Geometry check sheet. Reference: drawing and pictorial views, mm from the part's lowest x, y, z. A direction names the side the tool comes from. Give positions to 0.01 mm unless a question says otherwise; leave off trailing zeros. Write each loop counter-clockwise with the first axis right and the second up, starting at its lowest first coordinate (ties: lowest second). Pieces come first, ordered by that corner, then holes. Notation, with made-up numbers: M 29,25 L 46,25 A37 cw 46,61 Z; hole C 60,11.25 d8. An arc over 180 degrees is marked long. Write item = value, one per line. Start each with the question number.
1) Cross-section at D-D, the plane x = 11. Record the cut outline in (y, z), plus the area to 3 significant figures.
2) Cross-section at A-A, the plane x = 6.75. Record the cut outline in (y, z).
3) Cross-section at C-C, the plane y = 35.5. Record the cut outline in (x, z).
4) Access from +Z, -Z, +X, -X, +Y, -Y to the whole of each face (thin tool, end or side, straight path). Record for the marked faces 4 and 5.
5) Scan lines: line 1 along X through (y, z) = (33.5, 1.75); line 2 along Z through (x, y) = (5.75, 25); line 3 along Y through (x, z) = (9.25, 8.5). Record each from-to range of solid material in increasing order. Write a range as [from, to].
6) Mould release check, pull along X, two halves, no side actions. Record for the marked faces 1, 2 and 3: released by +X, released by -X, zero draft, split by the parting line, or undercut.
7) Cross-section at B-B, the plane z = 6.5. Record the cut outline in (x, y), plus the area to 3 significant figures.
8) Go/stop test with a flat-tipped pin: pin 1 (1 mm diameter, centred on x = 1.5, y = 10, fed in from +Z). Record where the tip stops, or that it passes through.
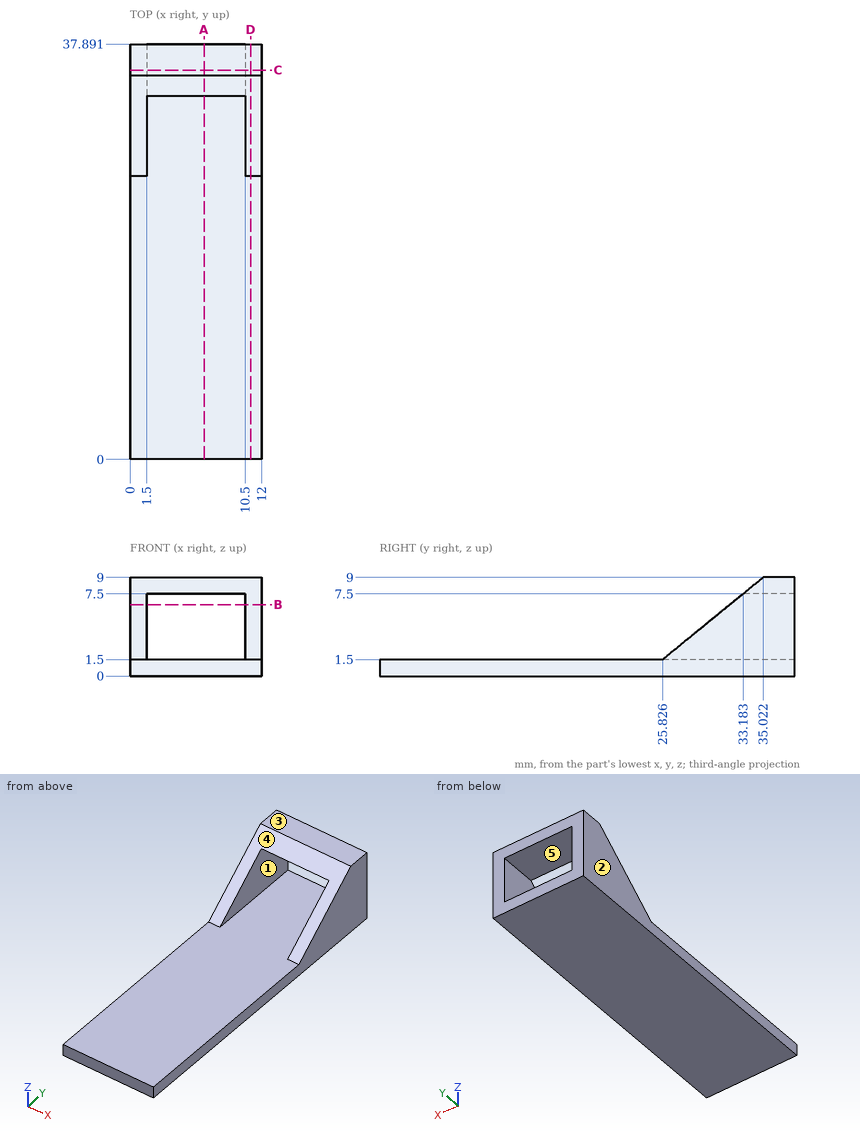
Reply:
q1.outline = M 0,0 L 37.89,0 L 37.89,9 L 35.02,9 L 25.83,1.5 L 0,1.5 Z
q1.area = 113 mm2
q2.outline = M 0,0 L 37.89,0 L 37.89,1.5 L 0,1.5 Z; M 33.18,7.5 L 37.89,7.5 L 37.89,9 L 35.02,9 Z
q3.outline = M 0,0 L 12,0 L 12,9 L 0,9 Z; hole M 1.5,1.5 L 10.5,1.5 L 10.5,7.5 L 1.5,7.5 Z
q4.face_4 = +Z, +X, -X, -Y
q4.face_5 = +Y, -Y
q5.line_1 = [0, 1.5], [10.5, 12]
q5.line_2 = [0, 1.5]
q5.line_3 = [34.41, 37.89]
q6.face_1 = undercut
q6.face_2 = released by -X
q6.face_3 = zero draft
q7.outline = M 0,31.96 L 1.5,31.96 L 1.5,37.89 L 0,37.89 Z; M 10.5,31.96 L 12,31.96 L 12,37.89 L 10.5,37.89 Z
q7.area = 17.8 mm2
q8.pin_1 = 1.5
